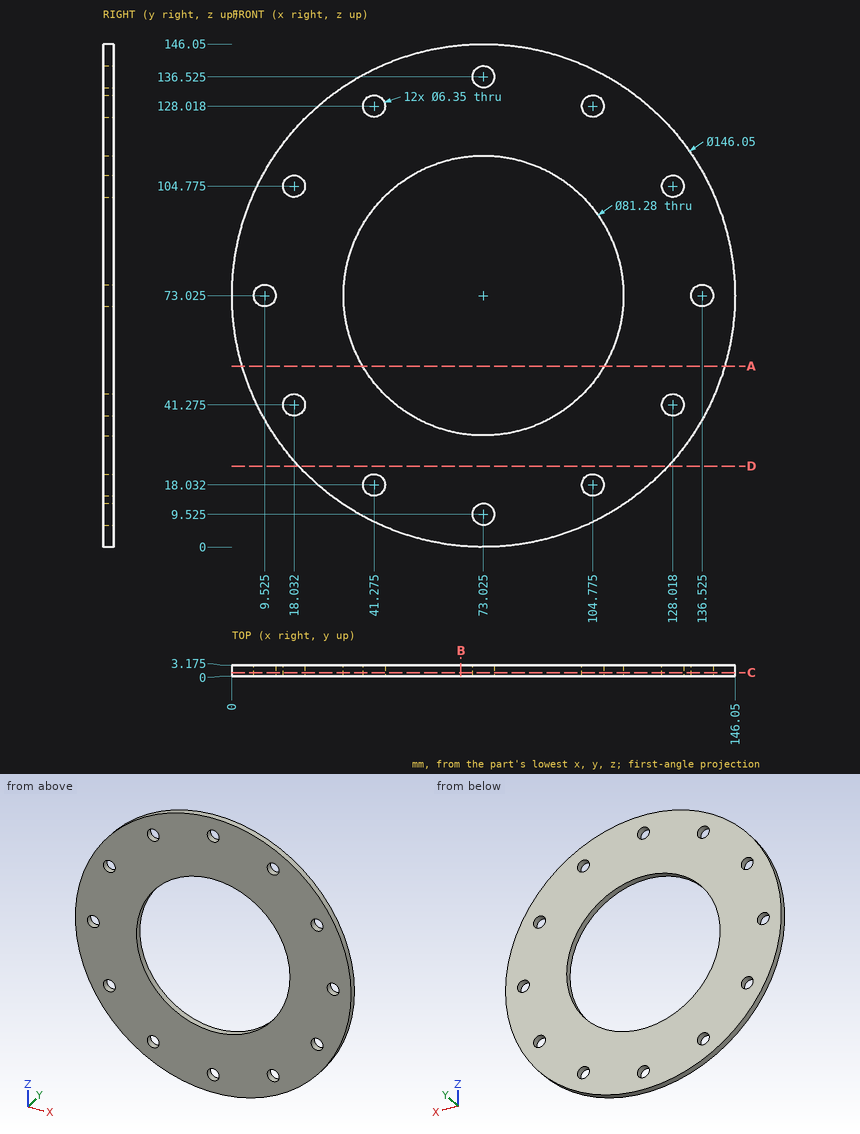
Could you check a few things on this drawing? It's one solid part, dimensions in mm from its lowest x, y, z. Coordinates: 2 decimals unless noted, no trailing zeros. Order: outer loops, then holes, each group sorted by start corner. A loop starts at its lowest first (then second) coordinate and runs counter-clockwise, first axis right, second up. Notation, with made-up numbers: M -27.75,72.5 L 12.25,72.5 A17 ccw 12.25,90.5 Z; hole C -38,46 d5. An arc over 180 degrees is marked long. Use one line per item in the form item = value. Start each with the question number.
1. Suppose I cut it at A-A on z = 52.5. Write out the boundary of the cut face in (x, y) (1 decimal).
2. For pin 1 (1.5 mm diameter, centred on y = 2, z = 30.5, fed in from +X); pin 2 (5 mm diameter, centred on x = 41.28, z = 128.02, fed in from +Y), each with a flat end and sliding along its axis, tell me the tip position at first contact or that it passes through.
3. Suppose I cut it at B-B on x = 66.5. Write out the boundary of the cut face in (y, z) (1 decimal).
4. Please list where these lines run through material, in increasing order: line 1 (X direction, y = 0.85, z = 106) (1 decimal); line 2 (Z direction, x = 127, y = 2.15) (1 decimal); line 3 (X direction, y = 1.25, z = 126.5) (1 decimal).
5. Suppose I cut it at D-D on z = 23.5. Write out the boundary of the cut face in (x, y) (1 decimal).
6. Suppose I cut it at C-C on y = 0.95. Count the separate pieces of the cut face and the enclosed holes in it, then the cut area to 3 significant figures.
Geometry says:
q1.outline = M 2.9,0 L 37.9,0 L 37.9,3.2 L 2.9,3.2 Z; M 108.1,0 L 143.1,0 L 143.1,3.2 L 108.1,3.2 Z
q2.pin_1 = 132.92
q2.pin_2 = through
q3.outline = M 0,0.3 L 3.2,0.3 L 3.2,32.9 L 0,32.9 Z; M 0,113.1 L 3.2,113.1 L 3.2,145.8 L 0,145.8 Z
q4.line_1 = 7.9 to 15.1, 21 to 49.3, 96.8 to 125.1, 130.9 to 138.2
q4.line_2 = 23.8 to 38.3, 44.3 to 101.8, 107.8 to 122.2
q4.line_3 = 23.3 to 38.5, 44.1 to 102, 107.6 to 122.8
q5.outline = M 19.4,0 L 126.7,0 L 126.7,3.2 L 19.4,3.2 Z
q6.separate_pieces = 1
q6.enclosed_holes = 13
q6.area = 11,200 mm^2
